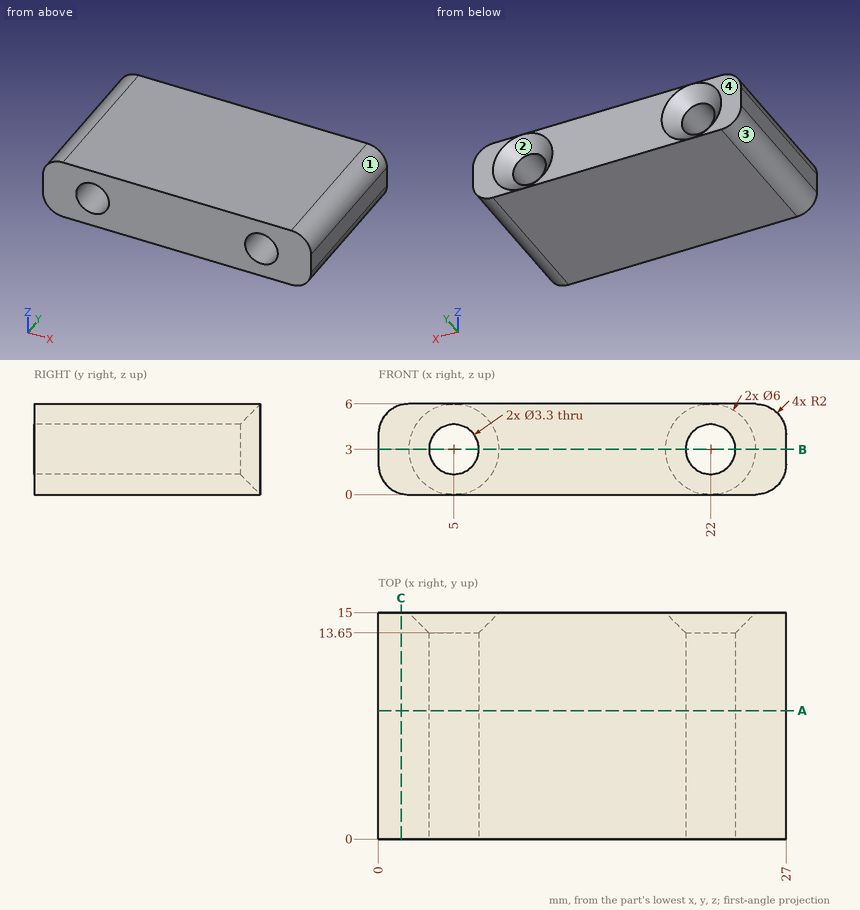
Design review of the part shown in the three views and the two pictorial views. Dimensions are in mm from the part's minimum x, y and z. Coordinates: 2 decimals unless noted, no trailing zeros. Order: outer loops, then holes, each group sorted by start corner. A loop starts at its lowest first (then second) coordinate and runs counter-clockwise, first axis right, second up.
Item 1: The part is to be moulded in two halves that separate along Z. For the marked faces 1, 2, 3 and 4, say which applies: pulls with the +Z half, pulls with the -Z half, needs draft (parallel to the pull), parting line crosses it, or undercut.
Item 2: For pin 1 Ø3 at (y, z) = (6, 1) entering from -X; pin 2 Ø2.5 at (x, z) = (22, 3) entering from -Y, all flat-tipped, find the tip position at first contact; note any pin that passes through.
Item 3: For line 1 (X direction, y = 5, z = 3); line 2 (Z direction, x = 5, y = 3.75); line 3 (X direction, y = 3.75, z = 4.45), list the stretches that pass through material, from the lowest coordinate up.
Item 4: Take a section at A-A, the plane y = 8.5. Write out the cut boundary in (x, z), then the cut area to 3 significant figures.
Item 5: Take a section at C-C, the plane x = 1.5. Write out the cut boundary in (y, z).
Item 6: Take a section at B-B, the plane z = 3. Write out the cut boundary in (x, y).
The answers:
1. face 1: pulls with the +Z half
1. face 2: undercut
1. face 3: pulls with the -Z half
1. face 4: needs draft
2. pin 1: stops at x = 0
2. pin 2: passes through
3. line 1: x = 0 to 3.35, 6.65 to 20.35, 23.65 to 27
3. line 2: z = 0 to 1.35, 4.65 to 6
3. line 3: x = 0.05 to 4.21, 5.79 to 21.21, 22.79 to 26.95
4. outline: (0, 2) arc R2 ccw to (2, 0) - (25, 0) arc R2 ccw to (27, 2) - (27, 4) arc R2 ccw to (25, 6) - (2, 6) arc R2 ccw to (0, 4) - close; hole circle Ø3.3 at (5, 3); hole circle Ø3.3 at (22, 3)
4. area: 141 mm2
5. outline: (0, 0.06) - (15, 0.06) - (15, 5.94) - (0, 5.94) - close
6. outline: (0, 0) - (3.35, 0) - (3.35, 13.65) - (2, 15) - (0, 15) - close; (6.65, 0) - (20.35, 0) - (20.35, 13.65) - (19, 15) - (8, 15) - (6.65, 13.65) - close; (23.65, 0) - (27, 0) - (27, 15) - (25, 15) - (23.65, 13.65) - close
